Drawing for the job (mm, zero at the part's lowest x, y, z). Coordinates: 2 decimals unless noted, no trailing zeros. Write each loop counter-clockwise with the first axis right and the second up, starting at its lowest first coordinate (ties: lowest second). Pieces come first, ordered by that corner, then holes. Notation, with made-up numbers: (6.5, -16.75) -> (28.5, -16.75) arc R17 cw to (28.5, -0.75) -> close; hole circle Ø9 at (8.5, 50.5). An arc over 180 degrees is marked (long way). Write item = value, one per line. Start each with the question number.
Q1. Band-saw the part on A-A, the plane z = 8.5. List the corners of the cut face in (x, y).
Q2. Band-saw the part on C-C, the plane x = 60. List the corners of the cut face in (y, z).
Q3. Probe line 1 (Y direction, x = 54.15, z = 2); line 2 (Y direction, x = 47, z = 8.5); line 3 (X direction, y = 62.5, z = 3.75). List the from-to ranges inside material, lowest first.
Q4. Band-saw the part on D-D, the plane x = 77. List the corners of the cut face in (y, z), plus the area to 3 significant figures.
Q5. Pull direction Y, two halves, no side cores. Call the marked faces 1, 2 and 3: released by +Y, released by -Y, zero draft, split by the parting line, or undercut.
Q6. Band-saw the part on B-B, the plane x = 48.5. List the corners of the cut face in (y, z).
Q7. Pin check, flat tip, straight feed: P1, Ø6, axis at y = 76.5, z = 8, coming from the +X side. Stop position of the tip, or through.
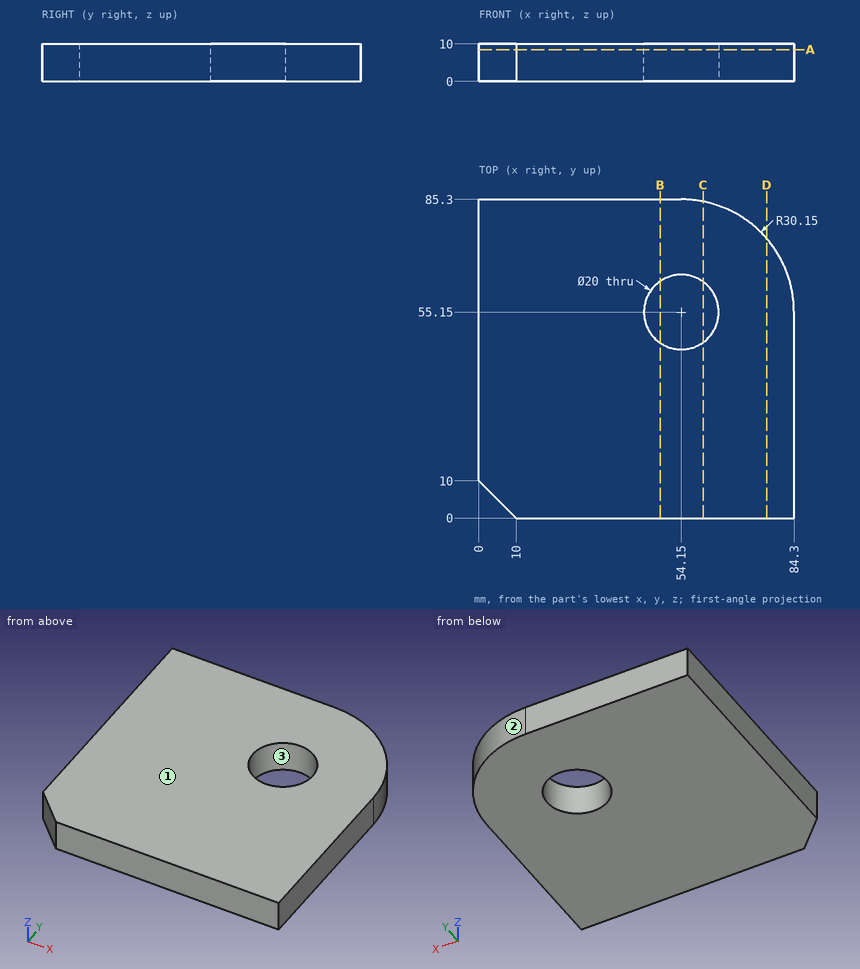
Ans:
q1.outline = (0, 10) -> (10, 0) -> (84.3, 0) -> (84.3, 55.15) arc R30.15 ccw to (54.15, 85.3) -> (0, 85.3) -> close; hole circle Ø20 at (54.15, 55.15)
q2.outline = (0, 0) -> (47.04, 0) -> (47.04, 10) -> (0, 10) -> close; (63.26, 0) -> (84.73, 0) -> (84.73, 10) -> (63.26, 10) -> close
q3.line_1 = 0 to 45.15, 65.15 to 85.3
q3.line_2 = 0 to 48.16, 62.14 to 85.3
q3.line_3 = 0 to 47.37, 60.93 to 83.39
q4.outline = (0, 0) -> (74.82, 0) -> (74.82, 10) -> (0, 10) -> close
q4.area = 748 mm2
q5.face_1 = zero draft
q5.face_2 = released by +Y
q5.face_3 = undercut
q6.outline = (0, 0) -> (46.9, 0) -> (46.9, 10) -> (0, 10) -> close; (63.4, 0) -> (85.3, 0) -> (85.3, 10) -> (63.4, 10) -> close
q7.P1 = 78.07
